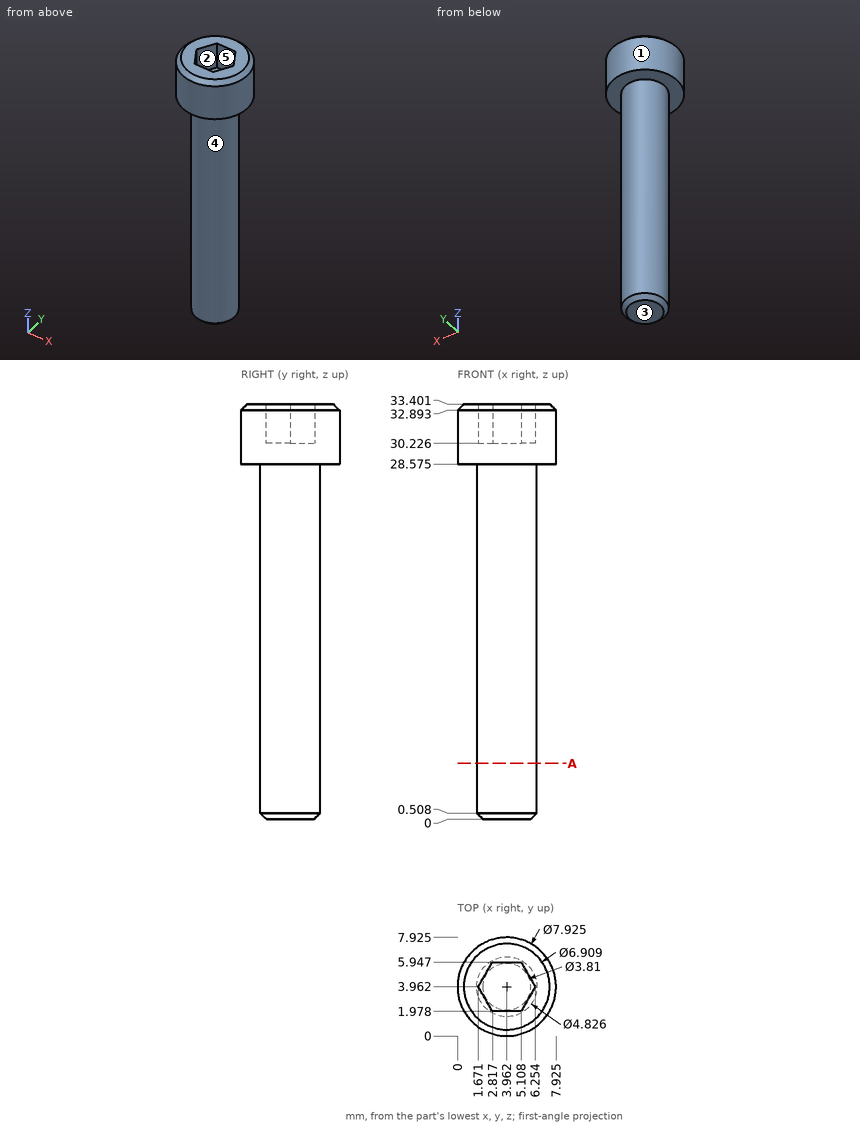
For this review, use the dimensioned drawing (mm, ordinates from the lowest corner) and the shaded views. A direction names the side the tool comes from. Coordinates: 2 decimals unless noted, no trailing zeros. Order: outer loops, then holes, each group sorted by start corner. A loop starts at its lowest first (then second) coordinate and runs counter-clockwise, first axis right, second up. Notation, with made-up numbers: (71, 28.5) - (116, 28.5) arc R15 ccw to (116, 46.5) - close; hole circle Ø2 at (78.5, 49.5). An arc over 180 degrees is marked (long way). Answer as a JSON object with one key per item and string values. Group by question number.
1. For probe 1 along Z at (x, y) = (5.25, 4); probe 2 along Z at (x, y) = (3.5, 7) (1 decimal); probe 3 along X at (y, z) = (6.25, 31), list the stretches that pass through material, from the lowest coordinate up.
2. Clearance check with flat-ended pins moving along their axes: P1, Ø1.2, axis at x = 3.5, y = 3, coming from the +Z side; P2, Ø3, axis at x = 3.5, z = 12.5, coming from the +Y side (1 decimal); P3, Ø0.7, axis at x = 4.5, z = 31, coming from the +Y side. State where each tip first meets the part, or that it passes through.
3. We need section A-A on z = 4.5. State the section outline as (x, y) points.
4. For the marked faces 4 and 5, list the 3-axis set-ups (+Z, -Z, +X, -X, +Y, -Y) from which the entire face can be reached by the end or side of a thin tool; tool diameter is ignored.
5. The part is to be moulded in two halves that separate along Y. For the marked faces 1, 2 and 3, say which applies: pulls with the +Y half, pulls with the -Y half, needs draft (parallel to the pull), parting line crosses it, or undercut.
Final values:
{
 "1": {"probe 1": "0 to 30.23", "probe 2": "28.6 to 33.4", "probe 3": "0.73 to 7.2"},
 "2": {"P1": "z = 30.23", "P2": "y = 6.4", "P3": "y = 7.92"},
 "3": {"outline": "circle Ø4.83 at (3.96, 3.96)"},
 "4": {"face 4": "-Z", "face 5": "+Z"},
 "5": {"face 1": "parting line crosses it", "face 2": "undercut", "face 3": "needs draft"}
}
